```python
from build123d import *

# Parameters (mm, degrees)
SKETCH1_R           = 75
SKETCH1_R_2         = 50
BOSS_EXTRUDE1_DEPTH = 2
CUT_EXTRUDE1_REACH  = 108.085
SKETCH2_W           = 5
SKETCH2_H           = 4
SKETCH4_W           = 3
SKETCH4_H           = 7
BOSS_EXTRUDE2_DEPTH = 10
SKETCH5_W           = 3
SKETCH5_H           = 7
BOSS_EXTRUDE3_DEPTH = 5
CIRPATTERN1_COUNT   = 2
CIRPATTERN1_ANGLE   = 135
CIRPATTERN2_COUNT   = 2
CIRPATTERN2_ANGLE   = 135
SKETCH6_R           = 5
BOSS_EXTRUDE4_DEPTH = 2
CIRPATTERN3_COUNT   = 3


with BuildPart() as part:
    # Sketch1 → Boss-Extrude1 (new body)
    with BuildSketch(Plane(origin=(0, 0, 0), x_dir=(1, 0, 0), z_dir=(0, 1, 0))):
        with Locations(Location((0, 0, 0), (0, 0, 270))):
            Circle(SKETCH1_R)
        with Locations(Location((0, 0, 0), (0, 0, 270))):
            Circle(SKETCH1_R_2, mode=Mode.SUBTRACT)
    extrude(amount=BOSS_EXTRUDE1_DEPTH)

    # Sketch2 → Cut-Extrude1 (cut, up to next)
    with BuildSketch(Plane(origin=(0, 2, 0), x_dir=(1, 0, 0), z_dir=(0, 1, 0)), mode=Mode.PRIVATE) as cut_extrude1_sk1:
        with Locations((0, 70)):
            Rectangle(SKETCH2_W, SKETCH2_H)
    cut_extrude1_tool1 = extrude(cut_extrude1_sk1.sketch, amount=-CUT_EXTRUDE1_REACH, mode=Mode.PRIVATE) & part.part
    add(cut_extrude1_tool1.solids().sort_by_distance((0, 2, -70))[0], mode=Mode.SUBTRACT)

    # Sketch4 → Boss-Extrude2 (add)
    with BuildSketch(Plane(origin=(0, 2, 0), x_dir=(1, 0, 0), z_dir=(0, 1, 0))):
        with Locations((3, 53.5)):
            Rectangle(SKETCH4_W, SKETCH4_H)
        with Locations((-3, 53.5)):
            Rectangle(SKETCH4_W, SKETCH4_H)
    boss_extrude2 = extrude(amount=BOSS_EXTRUDE2_DEPTH)

    # Sketch5 → Boss-Extrude3 (add)
    with BuildSketch(Plane(origin=(0, 2, 0), x_dir=(1, 0, 0), z_dir=(0, 1, 0))):
        with Locations((0, 53.5)):
            Rectangle(SKETCH5_W, SKETCH5_H)
    boss_extrude3 = extrude(amount=BOSS_EXTRUDE3_DEPTH)

    # CirPattern1: Boss-Extrude2, Boss-Extrude3 ×2 about axis
    cirpattern1_axis = Axis((0, 2, 0), (0, 1, 0))
    add([boss_extrude2.rotate(cirpattern1_axis, i * CIRPATTERN1_ANGLE / (CIRPATTERN1_COUNT - 1)) for i in range(1, CIRPATTERN1_COUNT)])
    add([boss_extrude3.rotate(cirpattern1_axis, i * CIRPATTERN1_ANGLE / (CIRPATTERN1_COUNT - 1)) for i in range(1, CIRPATTERN1_COUNT)])

    # CirPattern2: Boss-Extrude2, Boss-Extrude3 ×2 about axis
    cirpattern2_axis = Axis((0, 0, 0), (0, -1, 0))
    add([boss_extrude2.rotate(cirpattern2_axis, i * CIRPATTERN2_ANGLE / (CIRPATTERN2_COUNT - 1)) for i in range(1, CIRPATTERN2_COUNT)])
    add([boss_extrude3.rotate(cirpattern2_axis, i * CIRPATTERN2_ANGLE / (CIRPATTERN2_COUNT - 1)) for i in range(1, CIRPATTERN2_COUNT)])

    # Sketch6 → Boss-Extrude4 (add)
    with BuildSketch(Plane.XZ):
        with Locations((64.951905284, -37.5)):
            Circle(SKETCH6_R)
    boss_extrude4 = extrude(amount=-BOSS_EXTRUDE4_DEPTH)

    # CirPattern3: Boss-Extrude4 ×3 about axis
    cirpattern3_axis = Axis((0, 0, 0), (0, 1, 0))
    for i in range(1, CIRPATTERN3_COUNT):
        add(boss_extrude4.rotate(cirpattern3_axis, i * 360 / CIRPATTERN3_COUNT))


solid = part.part
```
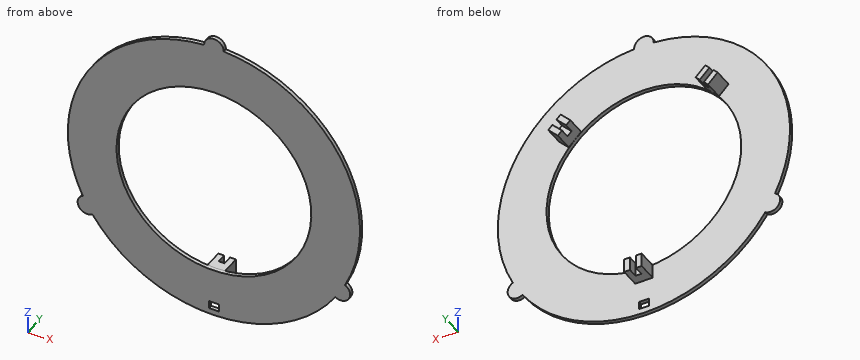
CAD build for the part. Positions are in the model's coordinates, mm. Round coordinates to 2 decimals unless told otherwise and drop trailing zeros. Order: outer loops, then holes, each group sorted by start corner. A loop starts at its lowest first (then second) coordinate and runs counter-clockwise, first axis right, second up. Notation, with made-up numbers: (-29.5, 31.5) - (10.5, 31.5) arc R15 ccw to (10.5, 39.5) - close; hole circle Ø10 at (28.25, 55.5). An arc over 180 degrees is marked (long way). Answer in a Markdown table with one row per item. Add a question column.
(1) Band-saw the part on D-D on x = 52.5. List the corners of the cut face in (y, z).
(2) Band-saw the part on C-C on z = 0. List the corners of the cut face in (x, y), and give its area (3 significant figures).
(3) Band-saw the part on B-B on z = 17.5. List the corners of the cut face in (x, y).
(4) Band-saw the part on A-A on y = 4. List the corners of the cut face in (x, z).
(5) Probe L1, parallel to X at y = 1.2, z = 0; L2, parallel to Z at x = -41, y = 1; L3, parallel to Y at x = -8, z = 62.5. List the from-to ranges inside material, lowest first. Write a range as [from, to].
(6) Drop flat-ended pins along their axis: pin 1 Ø2 at (x, y) = (-0.5, 1.5) entering from -Z; pin 2 Ø1.6 at (y, z) = (1, -69.5) entering from +X; pin 3 Ø2 at (y, z) = (8.5, -54) entering from +X; pin 4 Ø7 at (x, y) = (-2, 6.5) entering from -Z. Give the stop position or say it passes through.
Data:
| question | item | result |
|---|---|---|
| 1 | outline | (0, -53.56) - (2, -53.56) - (2, 53.56) - (0, 53.56) - close |
| 2 | outline | (-75, 0) - (-50, 0) - (-50, 2) - (-75, 2) - close; (50, 0) - (75, 0) - (75, 2) - (50, 2) - close |
| 2 | area | 100 mm^2 |
| 3 | outline | (-72.93, 0) - (-46.84, 0) - (-46.84, 2) - (-72.93, 2) - close; (46.84, 0) - (72.93, 0) - (72.93, 2) - (46.84, 2) - close |
| 4 | outline | (-43.49, 37.12) - (-38.54, 32.17) - (-32.17, 38.54) - (-37.12, 43.49) - close; (-4.5, -57) - (4.5, -57) - (4.5, -50) - (-4.5, -50) - close; (32.17, 38.54) - (38.54, 32.17) - (43.49, 37.12) - (37.12, 43.49) - close |
| 5 | L1 | x = [-75, -50], [50, 75] |
| 5 | L2 | z = [-62.8, -28.62], [28.62, 62.8] |
| 5 | L3 | y = [0, 2] |
| 6 | pin 1 | stops at z = -75 |
| 6 | pin 2 | stops at x = 30.09 |
| 6 | pin 3 | stops at x = 4.5 |
| 6 | pin 4 | stops at z = -57 |
